For this review, take the finished solid that the model builds, in its own axes (mm). A direction names the side the tool comes from. Round coordinates to 2 decimals unless told otherwise and drop trailing zeros. Order: outer loops, then holes, each group sorted by start corner. A loop starts at its lowest first (then second) coordinate and runs counter-clockwise, first axis right, second up. Notation, with made-up numbers: (-7, 22) -> (13, 22) arc R19 ccw to (13, 59) -> close; hole circle Ø5 at (36, 89). An arc over 180 degrees is marked (long way). Answer in a Markdown table with one row per item.
```python
from build123d import *

# Parameters (mm, degrees)
F0_W        = 58.166
F0_H        = 37.846
F1_DEPTH    = 2.54
F2_W        = 7.5946
F2_H        = 37.846
F3_DEPTH    = 2.54
F4_W        = 12.7
F4_H        = 0.635
F4_H_2      = 1.27
F5_DEPTH    = 2.54
F6_T1_DEPTH = 12.7
F7_W        = 4.445
F7_H        = 10.16
F8_DEPTH    = 4.445
F9_W        = 4.445
F9_H        = 5.08
F10_DEPTH   = 0.635
F12_DEPTH   = 0.635
F13_W       = 6.35
F13_H       = 6.35
F14_DEPTH   = 2.794


# Not quite as in the source:
# - a fillet or chamfer that OpenCascade refuses, or shapes differently, is made with other operations: its cross-section is extruded or revolved along the edge and cut away or added


with BuildPart() as f1:
    # F0 (on Top) → F1 (new body)
    with BuildSketch(Plane.XY):
        Rectangle(F0_W, F0_H)
    extrude(amount=F1_DEPTH)

    # F2 (on face) → F3 (join)
    with BuildSketch(Plane(origin=(0, 0, 0), x_dir=(1, 0, 0), z_dir=(0, 0, -1))):
        with Locations((25.2857, 0)):
            Rectangle(F2_W, F2_H)
    extrude(amount=F3_DEPTH)

    # F4 (on face) → F5 (join)
    with BuildSketch(Plane(origin=(-29.083, 0, 0), x_dir=(0, -1, 0), z_dir=(-1, 0, 0))):
        with Locations((0, -0.3175)):
            Rectangle(F4_W, F4_H)
        with Locations((0, 0.635)):
            Rectangle(F4_W, F4_H_2)
    extrude(amount=F5_DEPTH)

    # F6: fillet of radius 1.27 on 1 edges, made by hand

    # F6_s2 → F6_t1 (join)
    with BuildSketch(Plane.XZ.offset(-6.35)):
        with BuildLine():
            ThreePointArc((-27.9831477372, 0), (-28.6181477372, -0.1701477372), (-29.083, -0.635))
            Line((-29.083, -0.635), (-29.083, 0))
            Line((-29.083, 0), (-27.9831477372, 0))
        make_face()
    extrude(amount=F6_T1_DEPTH)

    # F7 (on face) → F8 (cut)
    with BuildSketch(Plane(origin=(0, 0, -2.54), x_dir=(1, 0, 0), z_dir=(0, 0, -1))):
        with Locations((25.5905, 0)):
            Rectangle(F7_W, F7_H)
    extrude(amount=-F8_DEPTH, mode=Mode.SUBTRACT)

    # F9 (on face) → F10 (cut)
    with BuildSketch(Plane(origin=(0, 0, -2.54), x_dir=(1, 0, 0), z_dir=(0, 0, -1))):
        with Locations((25.5905, 7.62)):
            Rectangle(F9_W, F9_H)
    extrude(amount=-F10_DEPTH, mode=Mode.SUBTRACT)

    # F11 (on face) → F12 (cut, through all)
    with BuildSketch(Plane(origin=(0, 0, 1.905), x_dir=(1, 0, 0), z_dir=(0, 0, -1))):
        with BuildLine():
            Line((25.527, -3.937), (25.781, -3.937))
            ThreePointArc((25.781, -3.937), (26.6790256121, -3.5650256121), (27.051, -2.667))
            Line((27.051, -2.667), (27.051, 2.667))
            ThreePointArc((27.051, 2.667), (26.6790256121, 3.5650256121), (25.781, 3.937))
            Line((25.781, 3.937), (25.527, 3.937))
            ThreePointArc((25.527, 3.937), (24.6289743879, 3.5650256121), (24.257, 2.667))
            Line((24.257, 2.667), (24.257, -2.667))
            ThreePointArc((24.257, -2.667), (24.6289743879, -3.5650256121), (25.527, -3.937))
        make_face()
    extrude(amount=-F12_DEPTH, mode=Mode.SUBTRACT)

    # F13 (on face) → F14 (cut)
    with BuildSketch(Plane(origin=(0, 0, -2.54), x_dir=(1, 0, 0), z_dir=(0, 0, -1))):
        with Locations((25.273, 15.113)):
            Rectangle(F13_W, F13_H)
    extrude(amount=-F14_DEPTH, mode=Mode.SUBTRACT)


solid = f1.part
```
Q1. Take a section at A-A, the plane y = 0.5. Write out the cut boundary in (x, z) (3 decimals).
Answer key:
| item | result |
|---|---|
| outline | (-31.623, -0.635) -> (-29.083, -0.635) arc R1.27 cw to (-27.983, 0) -> (21.488, 0) -> (21.488, -2.54) -> (23.368, -2.54) -> (23.368, 1.905) -> (24.257, 1.905) -> (24.257, 2.54) -> (-29.083, 2.54) -> (-29.083, 1.27) -> (-31.623, 1.27) -> close; (27.051, 1.905) -> (27.813, 1.905) -> (27.813, -2.54) -> (29.083, -2.54) -> (29.083, 2.54) -> (27.051, 2.54) -> close |
Q2. Take a section at C-C, the plane x = -5.5. Write out the cut boundary in (y, z), then the cut area to 3 significant figures.
Answer key:
| item | result |
|---|---|
| outline | (-18.92, 0) -> (18.92, 0) -> (18.92, 2.54) -> (-18.92, 2.54) -> close |
| area | 96.1 mm^2 |
Q3. Clearance check with flat-ended pins moving along their axes: pin 1 Ø0.8 at (y, z) = (-13.5, -0.5) entering from -X; pin 2 Ø2 at (x, y) = (-17, -12) entering from -Z; pin 3 Ø0.8 at (x, y) = (-30.5, 0) entering from +Z. State where each tip first meets the part, or that it passes through.
Answer key:
| item | result |
|---|---|
| pin 1 | stops at x = 21.49 |
| pin 2 | stops at z = 0 |
| pin 3 | stops at z = 1.27 |
Q4. Take a section at B-B, the plane y = -7.5. Write out the cut boundary in (x, z) (3 decimals), then the cut area to 3 significant figures.
Answer key:
| item | result |
|---|---|
| outline | (-29.083, 0) -> (21.488, 0) -> (21.488, -2.54) -> (23.368, -2.54) -> (23.368, -1.905) -> (27.813, -1.905) -> (27.813, -2.54) -> (29.083, -2.54) -> (29.083, 2.54) -> (-29.083, 2.54) -> close |
| area | 164 mm^2 |
Q5. Tool access review of faces 5 (the face through (24, 0, 1.905)), 6 (the face through (-28.61, 0.089, -0.166)), 7 (the face through (-30, 0, 1.27)), 8 (the face through (24.639, -3.575, 2.218)): name each direction out of +Z, -Z, +X, -X, +Y, -Y from which nothing blocks a thin tool from reaching the whole face with its end or side.
Answer key:
| item | result |
|---|---|
| face 5 | -Z |
| face 6 | -Z, +Y, -Y |
| face 7 | +Z, -X, +Y, -Y |
| face 8 | +Z, -Z |
Q6. The part is to be moulded in two halves that separate along X. For faces 1 (the face through (29.083, 0, 0)), 2 (the face through (-4, 0, 0)), 3 (the face through (0, 0, 2.54)), 4 (the face through (26.669, 3.575, 2.218)), say which applies: +X half, -X half, draft (parallel to the pull), parting line (faces both ways), or undercut.
Answer key:
| item | result |
|---|---|
| face 1 | +X half |
| face 2 | undercut |
| face 3 | draft |
| face 4 | undercut |
Q7. Take a section at D-D, the plane y = -14. Write out the cut boundary in (x, z).
Answer key:
| item | result |
|---|---|
| outline | (-29.08, 0) -> (21.49, 0) -> (21.49, -2.54) -> (22.1, -2.54) -> (22.1, 0.25) -> (28.45, 0.25) -> (28.45, -2.54) -> (29.08, -2.54) -> (29.08, 2.54) -> (-29.08, 2.54) -> close |
Q8. To check wall thickness, follow probe 1 along X at (y, z) = (3, 0.45); probe 2 along X at (y, z) = (3, -0.9); probe 3 along Z at (x, y) = (-5, 13). State the ranges of each line that lie inside material, in increasing order.
Answer key:
| item | result |
|---|---|
| probe 1 | x = -31.62 to 23.37, 27.81 to 29.08 |
| probe 2 | x = 21.49 to 23.37, 27.81 to 29.08 |
| probe 3 | z = 0 to 2.54 |
